CAD build for the part. Positions are in the model's coordinates, mm. Coordinates: 2 decimals unless noted, no trailing zeros. Loops run counter-clockwise (first coordinate to the right, second up) from the corner with the lowest first, then second, coordinate; pieces in that order, holes last. Notation, with made-up numbers: (50, -19) -> (95, -19) arc R10 ccw to (95, 0) -> close; hole circle Ø1 at (79, 41.25). An arc over 180 degrees is marked (long way). Write each question's results on one line, items separated by ' | '.
```python
from build123d import *

# Parameters (mm, degrees)
SKETCH1_R           = 2
BOSS_EXTRUDE2_DEPTH = 4
SKETCH2_R           = 3.5
CUT_EXTRUDE1_DEPTH  = 2
SKETCH3_R           = 3.5
CUT_EXTRUDE2_DEPTH  = 2


with BuildPart() as part:
    # Sketch1 → Boss-Extrude2 (new body)
    with BuildSketch(Plane.XY):
        with BuildLine():
            Line((29.982938543, -25.0000071), (29.982938543, 24.9999929))
            ThreePointArc((29.982938543, 24.9999929), (28.518472449, 28.535526806), (24.982938543, 29.9999929))
            Line((24.982938543, 29.9999929), (-25.017061457, 29.9999929))
            ThreePointArc((-25.017061457, 29.9999929), (-28.552595363, 28.535526806), (-30.017061457, 24.9999929))
            Line((-30.017061457, 24.9999929), (-30.017061457, -25.0000071))
            ThreePointArc((-30.017061457, -25.0000071), (-28.552595363, -28.535541006), (-25.017061457, -30.0000071))
            Line((-25.017061457, -30.0000071), (24.982938543, -30.0000071))
            ThreePointArc((24.982938543, -30.0000071), (28.518472449, -28.535541006), (29.982938543, -25.0000071))
        make_face()
        with Locations((-20.517061457, 20.4999929)):
            Circle(SKETCH1_R, mode=Mode.SUBTRACT)
        with Locations((-10.017061457, 0)):
            Circle(SKETCH1_R, mode=Mode.SUBTRACT)
        with Locations((-0.017061457, 0)):
            Circle(SKETCH1_R, mode=Mode.SUBTRACT)
        with Locations(Location((20.482938543, -20.5000071, 0), (0, 0, 180))):
            Circle(SKETCH1_R, mode=Mode.SUBTRACT)
        with Locations((0, 20.4999929)):
            Circle(SKETCH1_R, mode=Mode.SUBTRACT)
        with Locations((20.482938543, 20.4999929)):
            Circle(SKETCH1_R, mode=Mode.SUBTRACT)
        with Locations(Location((-20.517061457, -20.5000071, 0), (0, 0, 180))):
            Circle(SKETCH1_R, mode=Mode.SUBTRACT)
        with Locations((-0.017061457, 10)):
            Circle(SKETCH1_R, mode=Mode.SUBTRACT)
        with Locations((9.982938543, 0)):
            Circle(SKETCH1_R, mode=Mode.SUBTRACT)
        with Locations((-0.017061457, -10)):
            Circle(SKETCH1_R, mode=Mode.SUBTRACT)
        with Locations((20.5000071, 0)):
            Circle(SKETCH1_R, mode=Mode.SUBTRACT)
        with Locations((0, -20.5000071)):
            Circle(SKETCH1_R, mode=Mode.SUBTRACT)
        with Locations((-20.5, 0)):
            Circle(SKETCH1_R, mode=Mode.SUBTRACT)
    extrude(amount=BOSS_EXTRUDE2_DEPTH)

    # Sketch2 → Cut-Extrude1 (cut)
    with BuildSketch(Plane.XY.offset(4)):
        with Locations((-20.517061457, 20.4999929)):
            Circle(SKETCH2_R)
        with Locations((-20.517061457, -20.5000071)):
            Circle(SKETCH2_R)
        with Locations((20.482938543, -20.5000071)):
            Circle(SKETCH2_R)
        with Locations((20.482938543, 20.4999929)):
            Circle(SKETCH2_R)
    extrude(amount=-CUT_EXTRUDE1_DEPTH, mode=Mode.SUBTRACT)

    # Sketch3 → Cut-Extrude2 (cut)
    with BuildSketch(Plane(origin=(0, 0, 0), x_dir=(-1, 0, 0), z_dir=(0, 0, -1))):
        with Locations((-20.5000071, 0)):
            Circle(SKETCH3_R)
        with Locations((20.5, 0)):
            Circle(SKETCH3_R)
        with Locations((0, 20.4999929)):
            Circle(SKETCH3_R)
        with Locations((0, -20.5000071)):
            Circle(SKETCH3_R)
    extrude(amount=-CUT_EXTRUDE2_DEPTH, mode=Mode.SUBTRACT)


solid = part.part
```
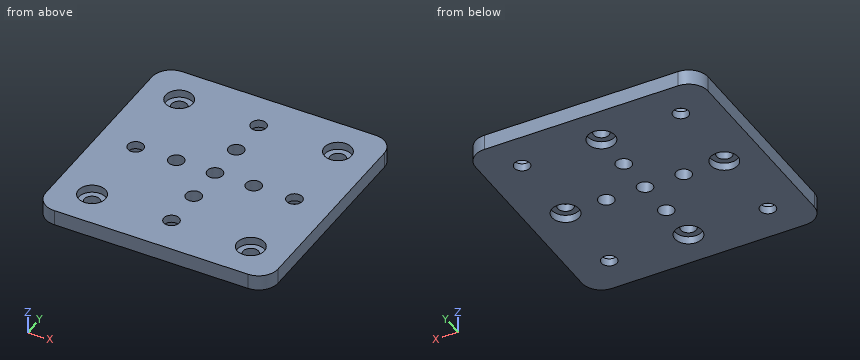
Q1. Cut at A-A on y = -10. Write the cut outline in (x, z), and give its area (3 significant figures).
Results are:
outline: (-30.02, 0) -> (-2.02, 0) -> (-2.02, 4) -> (-30.02, 4) -> close; (1.98, 0) -> (29.98, 0) -> (29.98, 4) -> (1.98, 4) -> close | area: 224 mm^2
Q2. Wall check: L1, parallel to Y at x = -20.5, z = 3.05; L2, parallel to Y at x = 0, z = 2.75; L3, parallel to Y at x = -20.5, z = 1.3. Give the ranges that are in metal, low to high. Write a range as from..to.
Results are:
L1: -30..-24, -17..-2, 2..17, 24..30 | L2: -30..-22.5, -18.5..-12, -8..-2, 2..8, 12..18.5, 22.5..30 | L3: -30..-22.5, -18.5..-3.5, 3.5..18.5, 22.5..30
Q3. Drop a flat-ended pin along its axis: pin 1 (6.5 mm diameter, centred on x = 0, y = 20.5, fed in from -Z). Give the stop position or say it passes through.
Results are:
pin 1: z = 2
Q4. Cut at B-B on z = 3.15. Give the number of separate pieces and of enclosed holes in the cut face, and give its area (3 significant figures).
Results are:
separate pieces: 1 | enclosed holes: 13 | area: 3,310 mm^2
